from build123d import *

# Parameters (mm, degrees)
SKETCH1_W           = 66.5
SKETCH1_H           = 27
SKETCH1_R           = 2
BOSS_EXTRUDE1_DEPTH = 1.6
SKETCH2_W           = 5.6
SKETCH2_H           = 7.1
BOSS_EXTRUDE2_DEPTH = 2.7
SKETCH3_W           = 51.4
SKETCH3_H           = 2.45
BOSS_EXTRUDE3_DEPTH = 8


with BuildPart() as part:
    # Sketch1 → Boss-Extrude1 (new body)
    with BuildSketch(Plane(origin=(0, 0, 0), x_dir=(1, 0, 0), z_dir=(0, 1, 0))):
        Rectangle(SKETCH1_W, SKETCH1_H)
        with Locations(Location((-30, 9, 0), (0, 0, 270))):
            Circle(SKETCH1_R, mode=Mode.SUBTRACT)
        with Locations(Location((-30, -9, 0), (0, 0, 270))):
            Circle(SKETCH1_R, mode=Mode.SUBTRACT)
        with Locations(Location((30, -9, 0), (0, 0, 270))):
            Circle(SKETCH1_R, mode=Mode.SUBTRACT)
        with Locations(Location((30, 9, 0), (0, 0, 270))):
            Circle(SKETCH1_R, mode=Mode.SUBTRACT)
    extrude(amount=BOSS_EXTRUDE1_DEPTH)

    # Sketch2 → Boss-Extrude2 (add)
    with BuildSketch(Plane(origin=(0, 1.6, 0), x_dir=(1, 0, 0), z_dir=(0, 1, 0))):
        with Locations((-31.45, 0)):
            Rectangle(SKETCH2_W, SKETCH2_H)
    extrude(amount=BOSS_EXTRUDE2_DEPTH)

    # Sketch3 → Boss-Extrude3 (add)
    with BuildSketch(Plane(origin=(0, 1.6, 0), x_dir=(1, 0, 0), z_dir=(0, 1, 0))):
        with Locations((0, 11.275)):
            Rectangle(SKETCH3_W, SKETCH3_H)
        with Locations((0, -11.275)):
            Rectangle(SKETCH3_W, SKETCH3_H)
    extrude(amount=BOSS_EXTRUDE3_DEPTH)


solid = part.part
The model under review builds one solid part; all positions refer to its coordinate system, in mm. A direction names the side the tool comes from. Round coordinates to 2 decimals unless told otherwise and drop trailing zeros. Write each loop counter-clockwise with the first axis right and the second up, starting at its lowest first coordinate (ties: lowest second). Pieces come first, ordered by that corner, then holes. Notation, with made-up numbers: (23.5, 84.25) - (39.5, 84.25) arc R24 ccw to (39.5, 115.25) - close; hole circle Ø4 at (0.25, 46). An arc over 180 degrees is marked (long way). One line per item, written item: value. Start each with the question number.
1. Consider section A-A on y = 3. Write out the cut boundary in (x, z), and give its area (3 significant figures).
2. The part is to be moulded in two halves that separate along X. For faces 1 (the face through (28, 1, 9)), 2 (the face through (-25.7, 6, -11)), 3 (the face through (-32, 1, 9)), 4 (the face through (0, 9.6, -11)), say which applies: released by +X, released by -X, zero draft, split by the parting line, or undercut.
3. Machinability: for faces 5 (the face through (-31, 3, -3.55)), 6 (the face through (0, 6, 12.5)), 7 (the face through (0, 6, -10.05)), 8 (the face through (-33.25, 1, 0)), 9 (the face through (-25.7, 6, 11)), which of the approach directions +Z, -Z, +X, -X, +Y, -Y give a long, thin tool a straight path to every point of the face, cutting with its end or side? Answer none if there is none.
4. Clearance check with flat-ended pins moving along their axes: P1, Ø3, axis at x = -30.5, z = 1.5, coming from the +Y side; P2, Ø0.5, axis at x = -34, z = 1.5, coming from the -Y side; P3, Ø1.3, axis at y = 1, z = -5, coming from the -X side. State where each tip first meets the part, or that it passes through.
5. Consider section B-B on x = 30. Write out the cut boundary in (y, z).
6. Consider section C-C on y = 8. Write out the cut boundary in (x, z).
7. Consider section D-D on z = -1. Write out the cut boundary in (x, y), and give its area (3 significant figures).
8. To check wall thickness, follow L1, parallel to X at y = 0.85, z = -9; L2, parallel to Z at x = -22.5, y = 1.75; L3, parallel to X at y = 0.5, z = 4. State the ranges of each line that lie inside material, in increasing order. Write a range as from..to.
Checks:
1. outline: (-34.25, -3.55) - (-28.65, -3.55) - (-28.65, 3.55) - (-34.25, 3.55) - close; (-25.7, -12.5) - (25.7, -12.5) - (25.7, -10.05) - (-25.7, -10.05) - close; (-25.7, 10.05) - (25.7, 10.05) - (25.7, 12.5) - (-25.7, 12.5) - close
1. area: 292 mm^2
2. face 1: undercut
2. face 2: released by -X
2. face 3: undercut
2. face 4: zero draft
3. face 5: -Z, +X, -X, +Y
3. face 6: +Z, +X, -X, +Y
3. face 7: +X, -X, +Y
3. face 8: +Z, -Z, -X, -Y
3. face 9: +Z, -Z, -X, +Y
4. P1: stops at y = 4.3
4. P2: stops at y = 1.6
4. P3: stops at x = -33.25
5. outline: (0, -13.5) - (1.6, -13.5) - (1.6, -11) - (0, -11) - close; (0, -7) - (1.6, -7) - (1.6, 7) - (0, 7) - close; (0, 11) - (1.6, 11) - (1.6, 13.5) - (0, 13.5) - close
6. outline: (-25.7, -12.5) - (25.7, -12.5) - (25.7, -10.05) - (-25.7, -10.05) - close; (-25.7, 10.05) - (25.7, 10.05) - (25.7, 12.5) - (-25.7, 12.5) - close
7. outline: (-34.25, 1.6) - (-33.25, 1.6) - (-33.25, 0) - (33.25, 0) - (33.25, 1.6) - (-28.65, 1.6) - (-28.65, 4.3) - (-34.25, 4.3) - close
7. area: 122 mm^2
8. L1: x = -33.25..-32, -28..28, 32..33.25
8. L2: z = -12.5..-10.05, 10.05..12.5
8. L3: x = -33.25..33.25
